```python
from build123d import *

# Parameters (mm, degrees)
F2_R = 2.53999


# Not quite as in the source:
# - a fillet or chamfer is up to 0.001 mm smaller than in the source, because OpenCascade refuses the exact size


with BuildPart() as f1:
    # F0 (on Front) → F1 (revolve)
    with BuildSketch(Plane.XZ):
        with BuildLine():
            Line((0, 17.78), (0, 0))
            Line((0, 0), (12.7, 0))
            Line((12.7, 0), (12.7, 10.16))
            ThreePointArc((12.7, 10.16), (11.9560512242, 11.9560512242), (10.16, 12.7))
            ThreePointArc((10.16, 12.7), (11.9560512242, 13.4439487758), (12.7, 15.24))
            Line((12.7, 15.24), (12.7, 17.78))
            Line((12.7, 17.78), (0, 17.78))
        make_face()
    revolve(axis=Axis((0, 0, 8.89), (0, 0, -1)))

    # F2 (radius 2.54 in the source; OpenCascade refuses exactly that, so slightly less here)
    f2_edges = [f1.edges().sort_by_distance(p)[0] for p in [
        (-12.7, 0, 17.78),
    ]]
    fillet(f2_edges, radius=F2_R)


solid = f1.part
```
CAD build for the part. Positions are in the model's coordinates, mm. Give positions to 0.01 mm unless a question says otherwise; leave off trailing zeros. Order: outer loops, then holes, each group sorted by start corner. A loop starts at its lowest first (then second) coordinate and runs counter-clockwise, first axis right, second up.
(1) Flat gauge pins, fed straight in: pin 1 (3 mm diameter, centred on y = -9.5, z = 7.5, fed in from -X); pin 2 (4 mm diameter, centred on x = -9.5, z = 2, fed in from +Y). Where does each tip first touch, or does it go through?
(2) Saw through at C-C, the plane z = 9.25. Give the cut face in (x, y).
(3) Drill centre lines: L1, parallel to Z at x = 11.25, y = -2; L2, parallel to Y at x = -0.25, z = 8.25; L3, parallel to Z at x = -11, y = -2. Where is each one in solid material? Low to high.
Results found:
1. pin 1: stops at x = -9.86
1. pin 2: stops at y = 10.25
2. outline: circle Ø25.4 at (0, 0)
3. L1: z = 0 to 12.36, 13.04 to 17.44
3. L2: y = -12.7 to 12.7
3. L3: z = 0 to 12.49, 12.91 to 17.57
